The listing builds one solid part. Answer for the finished solid, in the listing's coordinates (mm). A direction names the side the tool comes from. Round coordinates to 2 decimals unless told otherwise and drop trailing zeros. Write each loop counter-clockwise with the first axis right and the second up, starting at its lowest first coordinate (ties: lowest second). Pieces come first, ordered by that corner, then holes. Notation, with made-up numbers: M 70,-20.5 L 124,-20.5 A32 cw 124,18.5 Z; hole C 57,63.25 d5. An arc over 180 degrees is marked long. One line per item, written item: value. Start each with the question number.
(1) For a pull along Z with two mould halves and no side action, classify faces 1 (the cylindrical face through (4.93, -150.639, -71.167)), 2 (the flat face through (10, -152, -68)), 3 (the flat face through (4.93, -167.38, -49.63)) as released by +Z, released by -Z, zero draft, split by the parting line, or undercut.
(2) Given P1, Ø3, axis at x = 3.5, z = -63, coming from the -Y side; P2, Ø3, axis at x = 4.5, z = -69.5, coming from the +Y side; P3, Ø5, axis at x = 4.5, y = -136, coming from the -Z side; P4, Ø1.8, axis at y = -101.26, z = -69.78, coming from the -X side, each flat-ended and moving along its own axis, determine where each tip first touches the part or whether it passes through.
(3) Section B-B (y = -130) is taken. Determine the outline of the cut face in (x, z).
(4) Consider probe 1 along Y at (x, z) = (5.25, -42.5); probe 2 along Z at (x, y) = (8, -174); probe 3 along Y at (x, z) = (3.25, -47). Determine where each line is inside the solid, lowest interval first.
(5) Section C-C (x = 6) is taken. Determine the outline of the cut face in (y, z), plus the area to 3 significant figures.
(6) Section D-D (z = -104.5) is taken. Determine the outline of the cut face in (x, y).
(7) Section A-A (z = -35) is taken. Determine the outline of the cut face in (x, y), plus the area to 3 significant figures.
(8) For faces 4 (the flat face through (5, -105.314, -65)), 5 (the flat face through (5, -150, -74.781)), 6 (the flat face through (5, -127, -45.003)), determine the directions among +Z, -Z, +X, -X, +Y, -Y from which every point of the face is accessible in a straight line to the end or side of a thin tool.
```python
from build123d import *

# Parameters (mm, degrees)
SKETCH_7_R      = 1.5
EXTRUDE_2_DEPTH = 10


with BuildPart() as part:
    # 草图7 → 凸台-拉伸2 (new body)
    with BuildSketch(Plane(origin=(0, 0, 0), x_dir=(0, 0, -1), z_dir=(1, 0, 0))):
        Polygon((74.781222648, -105.314484454), (54.681222648, -105.314484454), (54.681222648, -146.014484454), (74.781222648, -146.014484454), (74.781222648, -153.864484454), (82.217885242, -173.050276706), (97.545045534, -202.471417533), (128.819415354, -228.557286652), (92.419152856, -214.512376165), (65.67699801, -187.583359255), (33.129337627, -146.599083723), (27.518646132, -119.704186977), (21.769974855, -92.147882993), (54.681222648, -75.517443579), (41.74198, -90.455051539), (49.731222648, -101.264484454), (54.681222648, -92.464484454), (65.67699801, -92.464484454), (74.781222648, -92.464484454), align=None)
        with Locations((69.781222648, -150.064484454)):
            Circle(SKETCH_7_R, mode=Mode.SUBTRACT)
        with Locations((59.681222648, -150.064484454)):
            Circle(SKETCH_7_R, mode=Mode.SUBTRACT)
        with Locations((69.781222648, -101.264484454)):
            Circle(SKETCH_7_R, mode=Mode.SUBTRACT)
        with Locations((59.681222648, -101.264484454)):
            Circle(SKETCH_7_R, mode=Mode.SUBTRACT)
        Polygon((85.031406178, -190.25046896), (71.623670801, -164.51374649), (59.47327237, -164.51374649), align=None, mode=Mode.SUBTRACT)
        Polygon((45.003171043, -144.573005818), (41.74198, -138.313009895), (32.111220405, -92.147882993), (45.003171043, -109.590672216), align=None, mode=Mode.SUBTRACT)
    extrude(amount=EXTRUDE_2_DEPTH)


solid = part.part
```
Recorded:
1. face 1: undercut
1. face 2: zero draft
1. face 3: released by +Z
2. P1: stops at y = -186.1
2. P2: stops at y = -92.46
2. P3: stops at z = -54.68
2. P4: passes through
3. outline: M 0,-54.68 L 10,-54.68 L 10,-45 L 0,-45 Z; M 0,-40.01 L 10,-40.01 L 10,-29.67 L 0,-29.67 Z
4. probe 1: y = -158.4 to -139.77, -106.2 to -91.48, -89.58 to -81.67
4. probe 2: z = -82.71 to -76.57, -68.89 to -54.89
4. probe 3: y = -164.07 to -97.57, -84.38 to -79.4
5. outline: M -228.56,-128.82 L -202.47,-97.55 L -173.05,-82.22 L -153.86,-74.78 L -146.01,-74.78 L -146.01,-54.68 L -105.31,-54.68 L -105.31,-74.78 L -92.46,-74.78 L -92.46,-54.68 L -101.26,-49.73 L -90.46,-41.74 L -75.52,-54.68 L -92.15,-21.77 L -146.6,-33.13 L -187.58,-65.68 L -214.51,-92.42 Z; hole M -190.25,-85.03 L -164.51,-71.62 L -164.51,-59.47 Z; hole C -150.06,-69.78 d3; hole C -150.06,-59.68 d3; hole M -144.57,-45 L -109.59,-45 L -92.15,-32.11 L -138.31,-41.74 Z; hole C -101.26,-69.78 d3; hole C -101.26,-59.68 d3
5. area: 3,340 mm2
6. outline: M 0,-219.17 L 10,-219.17 L 10,-208.27 L 0,-208.27 Z
7. outline: M 0,-148.95 L 10,-148.95 L 10,-106 L 0,-106 Z; M 0,-96.06 L 10,-96.06 L 10,-85.46 L 0,-85.46 Z
7. area: 536 mm2
8. face 4: -Z, +X, -X
8. face 5: -Z, +X, -X, +Y
8. face 6: +X, -X
